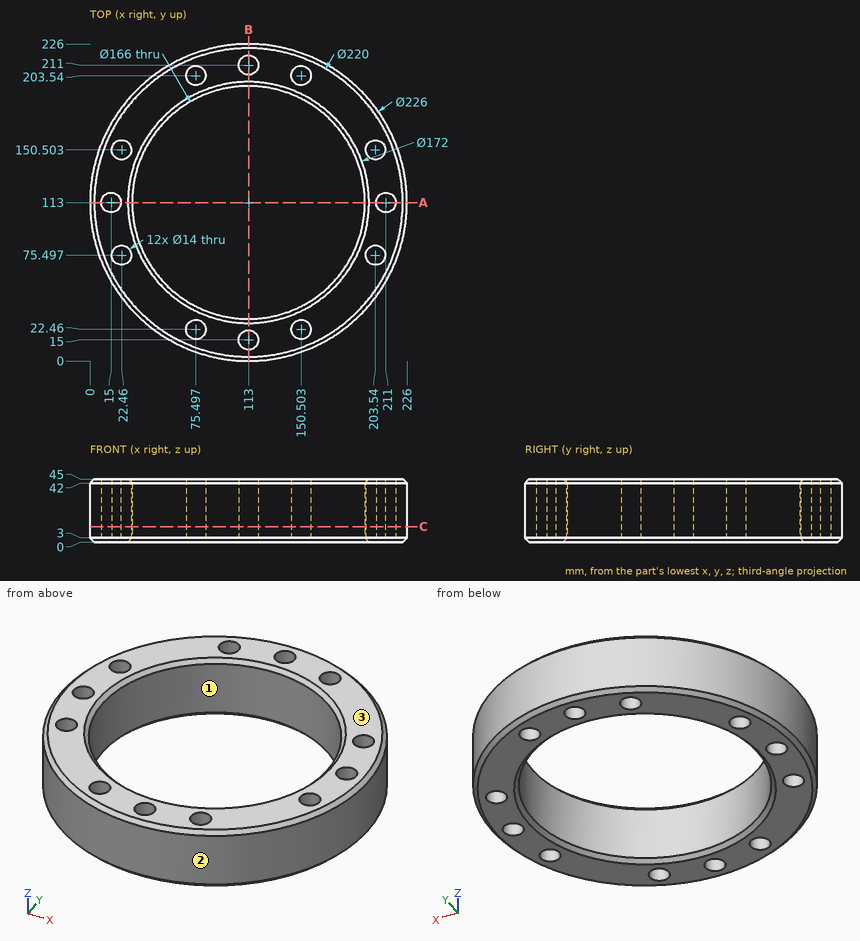
Drawing for the job (mm, zero at the part's lowest x, y, z). Round coordinates to 2 decimals unless told otherwise and drop trailing zeros. Order: outer loops, then holes, each group sorted by start corner. A loop starts at its lowest first (then second) coordinate and runs counter-clockwise, first axis right, second up. Notation, with made-up numbers: M 8.25,-24 L 52.25,-24 A20 cw 52.25,-13 Z; hole C 22.5,49.25 d7. An arc over 180 degrees is marked long. Use one line per item in the form item = value.
Q1. Two-plate mould, pull along Y, no slides. Class the marked faces 1, 2 and 3: +Y half, -Y half, draft (parallel to the pull), parting line (faces both ways), or undercut.
Recorded:
face_1 = undercut
face_2 = parting line
face_3 = draft
Q2. Saw through at A-A on y = 113. Give the cut face in (x, z), then the cut area to 3 significant figures.
Recorded:
outline = M 0,3 L 3,0 L 8,0 L 8,45 L 3,45 L 0,42 Z; M 22,0 L 27,0 L 30,3 L 30,42 L 27,45 L 22,45 Z; M 196,3 L 199,0 L 204,0 L 204,45 L 199,45 L 196,42 Z; M 218,0 L 223,0 L 226,3 L 226,42 L 223,45 L 218,45 Z
area = 1,400 mm^2
Q3. Probe L1, parallel to X at y = 20.5, z = 10.5 (1 decimal); L2, parallel to X at y = 75, z = 2; L3, parallel to Y at x = 147, z = 14.5. List the from-to ranges inside material, lowest first.
Recorded:
L1 = 48.1 to 68.8, 82.2 to 108.7, 117.3 to 143.8, 157.2 to 177.9
L2 = 7.64 to 15.48, 29.44 to 38.09, 187.91 to 196.56, 210.52 to 218.36
L3 = 5.24 to 16.4, 28.52 to 37.28, 188.72 to 197.48, 209.6 to 220.76
Q4. Flat gauge pins, fed straight in: P1, Ø11, axis at x = 203.54, y = 150.5, coming from the -Z side; P2, Ø1.5, axis at x = 183, y = 64.5, coming from the -Z side; P3, Ø1.5, axis at y = 146.5, z = 30.5, coming from the +X side; P4, Ø4, axis at x = 182.5, z = 9, coming from the +Y side. Where does each tip first touch, or does it go through?
Recorded:
P1 = through
P2 = 0.09
P3 = 221.15
P4 = 203.62
Q5. Saw through at C-C on z = 11. State how many separate pieces and enclosed holes the cut face has, then the cut area to 3 significant figures.
Recorded:
separate_pieces = 1
enclosed_holes = 13
area = 16,600 mm^2
